Part model, mm, in its own coordinate system. A direction names the side the tool comes from. Round coordinates to 2 decimals unless told otherwise and drop trailing zeros. Write each loop counter-clockwise with the first axis right and the second up, starting at its lowest first coordinate (ties: lowest second). Pieces come first, ordered by that corner, then holes. Notation, with made-up numbers: M -7,21 L 33,21 A18 cw 33,31 Z; hole C -28,3.5 d6. An arc over 180 degrees is marked long. Use a Markdown table: item, result. Add a question column.
1) Slice it at B-B on z = -19. Write the cut outline in (x, y).
2) Which spindle directions (+Z, -Z, +X, -X, +Y, -Y) get a long thin tool onto all of the face, cutting with end or side? Do faces 4 (the face through (0.241, 71.434, 22.306)), 5 (the face through (-15.61, 122.09, -20.36)). Say none if no direction does.
3) Slice it at A-A on z = -2. Write the cut outline in (x, y).
4) Slice it at C-C on x = 0. Give the number of separate pieces and of enclosed holes in the cut face, plus the area to 3 significant figures.
5) Drop flat-ended pins along their axis: P1, Ø3.5, axis at x = -15, y = 141, coming from the +Z side; P2, Ø7.5, axis at x = 13.5, y = 92, coming from the +Z side; P3, Ø1, axis at y = 166.5, z = 10, coming from the +X side; P4, Ø12, axis at x = 19.5, z = -3.5, coming from the -Y side. Give the stop position or say it passes through.
6) Wall check: probe 1 along X at (y, z) = (65, 0); probe 2 along Z at (x, y) = (-1, 111.5); probe 3 along Z at (x, y) = (-3.5, 157.5). Give the ranges that are in metal, low to high.
7) Two-plate mould, pull along Y, no slides. Class faces 1 (the face through (-0.24, 11.81, 22.31)), 2 (the face through (14, 211, 19.05)), 3 (the face through (12, 0, -19)): released by +Y, released by -Y, zero draft, split by the parting line, or undercut.
```python
from build123d import *

# Parameters (mm, degrees)
SKETCH1_R           = 25.654
SKETCH1_R_2         = 21.717
BOSS_EXTRUDE1_DEPTH = 247.65
CUT_EXTRUDE1_START  = 19.05
CUT_EXTRUDE1_DEPTH  = 12.7
LPATTERN1_START     = 19.05
LPATTERN1_DEPTH     = 6.604


# Read off the part's stored shape, not the designer's step: LPattern1
with BuildPart() as part:
    # Sketch1 → Boss-Extrude1 (new body)
    with BuildSketch(Plane(origin=(0, 0, 0), x_dir=(1, 0, 0), z_dir=(0, 1, 0))):
        with Locations(Location((0, 0, 0), (0, 0, 270))):
            Circle(SKETCH1_R)
        with Locations(Location((0, 0, 0), (0, 0, 270))):
            Circle(SKETCH1_R_2, mode=Mode.SUBTRACT)
    extrude(amount=BOSS_EXTRUDE1_DEPTH)

    # Sketch2 → Cut-Extrude1 (cut)
    with BuildSketch(Plane.XY.offset(CUT_EXTRUDE1_START)):
        Polygon((-28.03525, 216.65249706), (-25.654, 212.528051074), (28.03525, 243.525554014), (25.654, 247.65), align=None)
    extrude(amount=CUT_EXTRUDE1_DEPTH, mode=Mode.SUBTRACT)

    # LPattern1 outline → LPattern1 (cut)
    with BuildSketch(Plane.XY.offset(LPATTERN1_START)):
        Polygon((17.182119078, 229.296757269), (-17.182119078, 209.456555119), (-19, 208.407001079), (-19, 202.907739765), (-17.182119078, 203.957293805), (17.182119078, 223.797495955), (19, 224.847049995), (19, 230.346311309), align=None)
        Polygon((-17.182119078, 195.994555119), (-19, 194.945001079), (-19, 189.445739765), (-17.182119078, 190.495293805), (17.182119078, 210.335495955), (19, 211.385049995), (19, 216.884311309), (17.182119078, 215.834757269), align=None)
        Polygon((-17.182119078, 182.532555119), (-19, 181.483001079), (-19, 175.983739765), (-17.182119078, 177.033293805), (17.182119078, 196.873495955), (19, 197.923049995), (19, 203.422311309), (17.182119078, 202.372757269), align=None)
        Polygon((-17.182119078, 169.070555119), (-19, 168.021001079), (-19, 162.521739765), (-17.182119078, 163.571293805), (17.182119078, 183.411495955), (19, 184.461049995), (19, 189.960311309), (17.182119078, 188.910757269), align=None)
        Polygon((-17.182119078, 155.608555119), (-19, 154.559001079), (-19, 149.059739765), (-17.182119078, 150.109293805), (17.182119078, 169.949495955), (19, 170.999049995), (19, 176.498311309), (17.182119078, 175.448757269), align=None)
        Polygon((-17.182119078, 142.146555119), (-19, 141.097001079), (-19, 135.597739765), (-17.182119078, 136.647293805), (17.182119078, 156.487495955), (19, 157.537049995), (19, 163.036311309), (17.182119078, 161.986757269), align=None)
        Polygon((-17.182119078, 128.684555119), (-19, 127.635001079), (-19, 122.135739765), (-17.182119078, 123.185293805), (17.182119078, 143.025495955), (19, 144.075049995), (19, 149.574311309), (17.182119078, 148.524757269), align=None)
        Polygon((-17.182119078, 115.222555119), (-19, 114.173001079), (-19, 108.673739765), (-17.182119078, 109.723293805), (17.182119078, 129.563495955), (19, 130.613049995), (19, 136.112311309), (17.182119078, 135.062757269), align=None)
        Polygon((-17.182119078, 101.760555119), (-19, 100.711001079), (-19, 95.211739765), (-17.182119078, 96.261293805), (17.182119078, 116.101495955), (19, 117.151049995), (19, 122.650311309), (17.182119078, 121.600757269), align=None)
        Polygon((-17.182119078, 88.298555119), (-19, 87.249001079), (-19, 81.749739765), (-17.182119078, 82.799293805), (17.182119078, 102.639495955), (19, 103.689049995), (19, 109.188311309), (17.182119078, 108.138757269), align=None)
        Polygon((-17.182119078, 74.836555119), (-19, 73.787001079), (-19, 68.287739765), (-17.182119078, 69.337293805), (17.182119078, 89.177495955), (19, 90.227049995), (19, 95.726311309), (17.182119078, 94.676757269), align=None)
        Polygon((-17.182119078, 61.374555119), (-19, 60.325001079), (-19, 54.825739765), (-17.182119078, 55.875293805), (17.182119078, 75.715495955), (19, 76.765049995), (19, 82.264311309), (17.182119078, 81.214757269), align=None)
        Polygon((-17.182119078, 47.912555119), (-19, 46.863001079), (-19, 41.363739765), (-17.182119078, 42.413293805), (17.182119078, 62.253495955), (19, 63.303049995), (19, 68.802311309), (17.182119078, 67.752757269), align=None)
        Polygon((-17.182119078, 34.450555119), (-19, 33.401001079), (-19, 27.901739765), (-17.182119078, 28.951293805), (17.182119078, 48.791495955), (19, 49.841049995), (19, 55.340311309), (17.182119078, 54.290757269), align=None)
        Polygon((-17.182119078, 20.988555119), (-19, 19.939001079), (-19, 14.439739765), (-17.182119078, 15.489293805), (17.182119078, 35.329495955), (19, 36.379049995), (19, 41.878311309), (17.182119078, 40.828757269), align=None)
        Polygon((-17.182119078, 7.526555119), (-19, 6.477001079), (-19, 1), (-18.961444143, 1), (-17.182119078, 2.027293805), (17.182119078, 21.867495955), (19, 22.917049995), (19, 28.416311309), (17.182119078, 27.366757269), align=None)
    extrude(amount=LPATTERN1_DEPTH, mode=Mode.SUBTRACT)


solid = part.part
```
Entries:
| question | item | result |
|---|---|---|
| 1 | outline | M -17.24,0 L -10.52,0 L -10.52,247.65 L -17.24,247.65 Z; M 10.52,0 L 17.24,0 L 17.24,247.65 L 10.52,247.65 Z |
| 2 | face 4 | +Z |
| 2 | face 5 | +Y, -Y |
| 3 | outline | M -25.58,0 L -21.62,0 L -21.62,247.65 L -25.58,247.65 Z; M 21.62,0 L 25.58,0 L 25.58,247.65 L 21.62,247.65 Z |
| 4 | separate pieces | 19 |
| 4 | enclosed holes | 0 |
| 4 | area | 1,580 mm^2 |
| 5 | P1 | stops at z = 19.05 |
| 5 | P2 | stops at z = 23.73 |
| 5 | P3 | stops at x = 23.83 |
| 5 | P4 | stops at y = 0 |
| 6 | probe 1 | x = -25.65 to -21.72, 21.72 to 25.65 |
| 6 | probe 2 | z = -25.63 to -21.69, 21.69 to 25.63 |
| 6 | probe 3 | z = -25.41 to -21.43, 21.43 to 25.41 |
| 7 | face 1 | undercut |
| 7 | face 2 | undercut |
| 7 | face 3 | released by -Y |
